Could you check a few things on this drawing? It's one solid part, dimensions in mm from its lowest x, y, z. Give positions to 0.01 mm unless a question says otherwise; leave off trailing zeros. Order: outer loops, then holes, each group sorted by start corner. A loop starts at its lowest first (then second) coordinate and runs counter-clockwise, first axis right, second up. Notation, with made-up numbers: (82, 14) - (128, 14) arc R25 ccw to (128, 39) - close; hole circle Ø1 at (26, 66.25). An arc over 180 degrees is marked (long way). Put each result on its own line as item: value.
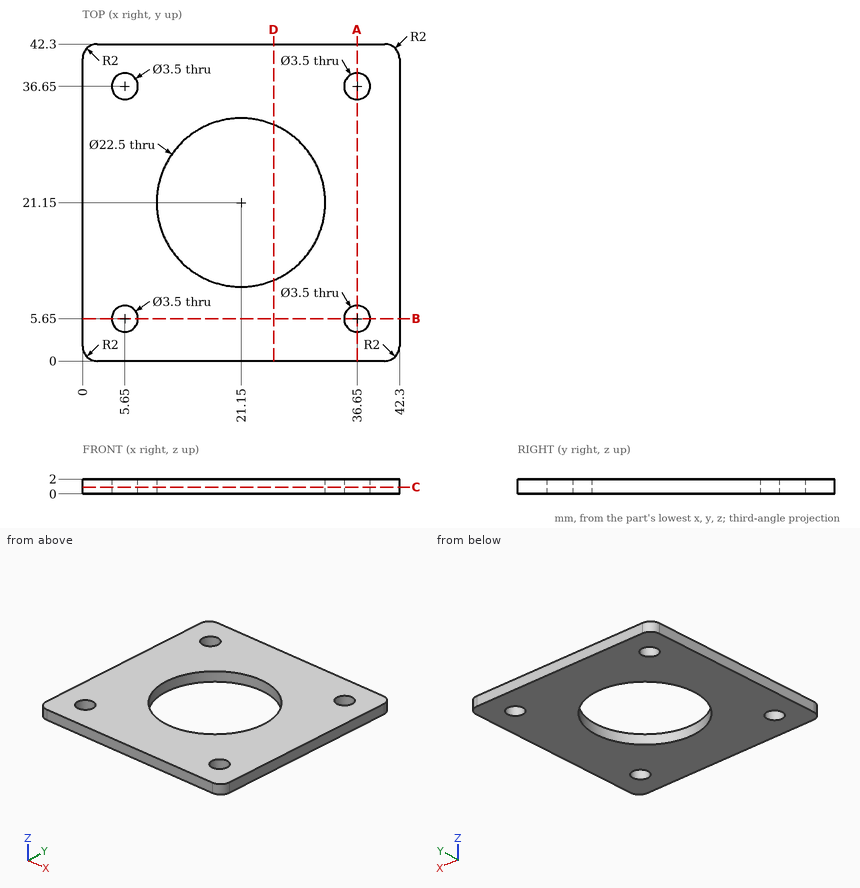
1) If I drill on line 1 (Y direction, x = 5.65, z = 1.2); line 2 (Y direction, x = 21.15, z = 1.45); line 3 (X direction, y = 5, z = 1.9), over which ranges is the centre line in solid material (lowest first)? Write a range as [from, to].
Filled in:
line 1: y = [0, 3.9], [7.4, 34.9], [38.4, 42.3]
line 2: y = [0, 9.9], [32.4, 42.3]
line 3: x = [0, 4.03], [7.27, 35.03], [38.27, 42.3]
2) Suppose I cut it at C-C, the plane z = 0.9. List the corners of the cut face in (x, y) for me, and give its area (3 significant figures).
Filled in:
outline: (0, 2) arc R2 ccw to (2, 0) - (40.3, 0) arc R2 ccw to (42.3, 2) - (42.3, 40.3) arc R2 ccw to (40.3, 42.3) - (2, 42.3) arc R2 ccw to (0, 40.3) - close; hole circle Ø3.5 at (5.65, 5.65); hole circle Ø3.5 at (5.65, 36.65); hole circle Ø22.5 at (21.15, 21.15); hole circle Ø3.5 at (36.65, 5.65); hole circle Ø3.5 at (36.65, 36.65)
area: 1,350 mm^2
3) Suppose I cut it at A-A, the plane x = 36.65. List the corners of the cut face in (y, z) for me.
Filled in:
outline: (0, 0) - (3.9, 0) - (3.9, 2) - (0, 2) - close; (7.4, 0) - (34.9, 0) - (34.9, 2) - (7.4, 2) - close; (38.4, 0) - (42.3, 0) - (42.3, 2) - (38.4, 2) - close
4) Suppose I cut it at D-D, the plane x = 25.5. List the corners of the cut face in (y, z) for me.
Filled in:
outline: (0, 0) - (10.78, 0) - (10.78, 2) - (0, 2) - close; (31.52, 0) - (42.3, 0) - (42.3, 2) - (31.52, 2) - close
